from build123d import *

# Parameters (mm, degrees)
SKETCH1_R           = 11
SKETCH1_R_2         = 8
BOSS_EXTRUDE1_DEPTH = 10
SKETCH1_5_R         = 11
BOSS_EXTRUDE3_DEPTH = 5
FILLET2_R           = 1
FILLET3_R           = 1


with BuildPart() as part:
    # Sketch1 → Boss-Extrude1 (new, symmetric)
    with BuildSketch(Plane.XY):
        Circle(SKETCH1_R)
        Circle(SKETCH1_R_2, mode=Mode.SUBTRACT)
    extrude(amount=BOSS_EXTRUDE1_DEPTH, both=True)

    # Sketch1_5 → Boss-Extrude3 (add, symmetric)
    with BuildSketch(Plane.XY):
        with BuildLine():
            ThreePointArc((14.784609691, 12), (13.338075004, 9.857677434), (10.810393031, 10.398817362))
            ThreePointArc((10.810393031, 10.398817362), (10.606601718, 10.606601718), (10.398817362, 10.810393031))
            ThreePointArc((10.398817362, 10.810393031), (9.857677434, 13.338075004), (12, 14.784609691))
            ThreePointArc((12, 14.784609691), (17.795554958, 19.23169542), (15, 25.980762114))
            ThreePointArc((15, 25.980762114), (0, 30), (-15, 25.980762114))
            ThreePointArc((-15, 25.980762114), (-17.795554958, 19.23169542), (-12, 14.784609691))
            ThreePointArc((-12, 14.784609691), (-9.857677434, 13.338075004), (-10.398817362, 10.810393031))
            ThreePointArc((-10.398817362, 10.810393031), (-10.606601718, 10.606601718), (-10.810393031, 10.398817362))
            ThreePointArc((-10.810393031, 10.398817362), (-13.338075004, 9.857677434), (-14.784609691, 12))
            ThreePointArc((-14.784609691, 12), (-19.23169542, 17.795554958), (-25.980762114, 15))
            ThreePointArc((-25.980762114, 15), (-30, 0), (-25.980762114, -15))
            ThreePointArc((-25.980762114, -15), (-19.23169542, -17.795554958), (-14.784609691, -12))
            ThreePointArc((-14.784609691, -12), (-13.338075004, -9.857677434), (-10.810393031, -10.398817362))
            ThreePointArc((-10.810393031, -10.398817362), (-10.606601718, -10.606601718), (-10.398817362, -10.810393031))
            ThreePointArc((-10.398817362, -10.810393031), (-9.857677434, -13.338075004), (-12, -14.784609691))
            ThreePointArc((-12, -14.784609691), (-17.795554958, -19.23169542), (-15, -25.980762114))
            ThreePointArc((-15, -25.980762114), (0, -30), (15, -25.980762114))
            ThreePointArc((15, -25.980762114), (17.795554958, -19.23169542), (12, -14.784609691))
            ThreePointArc((12, -14.784609691), (9.857677434, -13.338075004), (10.398817362, -10.810393031))
            ThreePointArc((10.398817362, -10.810393031), (10.606601718, -10.606601718), (10.810393031, -10.398817362))
            ThreePointArc((10.810393031, -10.398817362), (13.338075004, -9.857677434), (14.784609691, -12))
            ThreePointArc((14.784609691, -12), (19.23169542, -17.795554958), (25.980762114, -15))
            ThreePointArc((25.980762114, -15), (30, 0), (25.980762114, 15))
            ThreePointArc((25.980762114, 15), (19.23169542, 17.795554958), (14.784609691, 12))
        make_face()
        Circle(SKETCH1_5_R, mode=Mode.SUBTRACT)
        with BuildLine():
            ThreePointArc((-13.5, 23.382685902), (-14.598076211, 19.284609691), (-10.5, 18.186533479))
            ThreePointArc((-10.5, 18.186533479), (0, 21), (10.5, 18.186533479))
            ThreePointArc((10.5, 18.186533479), (14.598076211, 19.284609691), (13.5, 23.382685902))
            ThreePointArc((13.5, 23.382685902), (0, 27), (-13.5, 23.382685902))
        make_face(mode=Mode.SUBTRACT)
        with BuildLine():
            ThreePointArc((23.382685902, 13.5), (19.284609691, 14.598076211), (18.186533479, 10.5))
            ThreePointArc((18.186533479, 10.5), (21, 0), (18.186533479, -10.5))
            ThreePointArc((18.186533479, -10.5), (19.284609691, -14.598076211), (23.382685902, -13.5))
            ThreePointArc((23.382685902, -13.5), (27, 0), (23.382685902, 13.5))
        make_face(mode=Mode.SUBTRACT)
        with BuildLine():
            ThreePointArc((13.5, -23.382685902), (14.598076211, -19.284609691), (10.5, -18.186533479))
            ThreePointArc((10.5, -18.186533479), (0, -21), (-10.5, -18.186533479))
            ThreePointArc((-10.5, -18.186533479), (-14.598076211, -19.284609691), (-13.5, -23.382685902))
            ThreePointArc((-13.5, -23.382685902), (0, -27), (13.5, -23.382685902))
        make_face(mode=Mode.SUBTRACT)
        with BuildLine():
            ThreePointArc((-23.382685902, -13.5), (-19.284609691, -14.598076211), (-18.186533479, -10.5))
            ThreePointArc((-18.186533479, -10.5), (-21, 0), (-18.186533479, 10.5))
            ThreePointArc((-18.186533479, 10.5), (-19.284609691, 14.598076211), (-23.382685902, 13.5))
            ThreePointArc((-23.382685902, 13.5), (-27, 0), (-23.382685902, -13.5))
        make_face(mode=Mode.SUBTRACT)
    extrude(amount=BOSS_EXTRUDE3_DEPTH, both=True)

    # Fillet2
    fillet2_edges = [part.edges().sort_by_distance(p)[0] for p in [
        (-11, 0, -10),
        (-8, 0, -10),
    ]]
    fillet(fillet2_edges, radius=FILLET2_R)

    # Fillet3
    fillet3_edges = [part.edges().sort_by_distance(p)[0] for p in [
        (-11, 0, -5),
    ]]
    fillet(fillet3_edges, radius=FILLET3_R)


solid = part.part
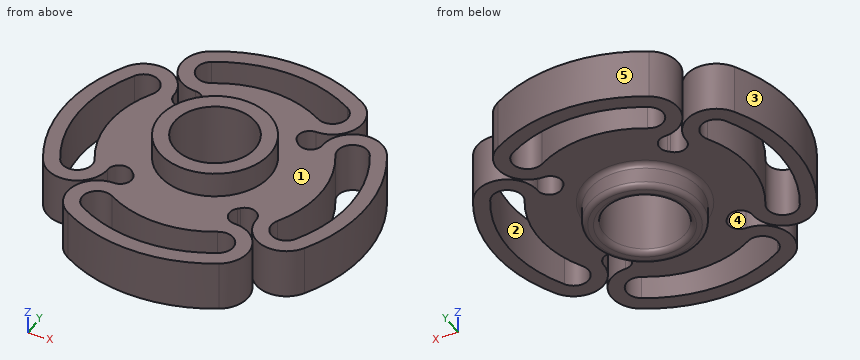
The model under review builds one solid part; all positions refer to its coordinate system, in mm. Face numbers are marked on the shaded views. A direction names the side the tool comes from. Round coordinates to 2 decimals unless told otherwise and drop trailing zeros. Order: outer loops, then holes, each group sorted by start corner. A loop starts at its lowest first (then second) coordinate and runs counter-clockwise, first axis right, second up. Notation, with made-up numbers: (68, 21) - (121, 21) arc R23 cw to (121, 42) - close; hole circle Ø6 at (-35, 36). An arc over 180 degrees is marked (long way). Use one line per item in the form item = value.
Q1. Mouldability with a two-part tool opening along X and no side actions: class the marked faces 3, 4 and 5 as pulls with the +X half, pulls with the -X half, needs draft (parallel to the pull), parting line crosses it, or undercut.
Response values:
face_3 = pulls with the -X half
face_4 = undercut
face_5 = parting line crosses it
Q2. Add section A-A on x = 0. Give the number of separate pieces and of enclosed holes in the cut face, then the cut area to 3 significant figures.
Response values:
separate_pieces = 4
enclosed_holes = 0
area = 380 mm^2
Q3. Clearance check with flat-ended pins moving along their axes: P1, Ø1.5, axis at x = 12, z = 7, coming from the -Y side; P2, Ø8, axis at x = 8.5, z = -6.5, coming from the +Y side; P3, Ø3, axis at x = 6, z = -4, coming from the -Y side; P4, Ø10, axis at y = -14.5, z = 7.5, coming from the +X side. State where each tip first meets the part, or that it passes through.
Response values:
P1 = through
P2 = 29.61
P3 = -29.66
P4 = 28.22
Q4. Add section C-C on x = 16.5. Give the boundary of the cut face in (y, z), then the cut area to 3 significant figures.
Response values:
outline = (-24.75, -5) - (-16.82, -5) - (-16.82, 5) - (-24.75, 5) - close; (-16.2, -5) - (16.2, -5) - (16.2, 5) - (-16.2, 5) - close; (16.82, -5) - (24.75, -5) - (24.75, 5) - (16.82, 5) - close
area = 483 mm^2
Q5. To check wall thickness, follow line 1 (Y direction, x = 0, z = -4); line 2 (Y direction, x = 3, z = 1.75); line 3 (Y direction, x = 9, z = 2.75). State the ranges of each line that lie inside material, in increasing order.
Response values:
line_1 = -30 to -27, -21 to -8, 8 to 21, 27 to 30
line_2 = -29.85 to -26.83, -20.78 to -7.42, 7.42 to 20.78, 26.83 to 29.85
line_3 = -28.62 to -25.46, -18.97 to 18.97, 25.46 to 28.62
Q6. Tool access review of the marked faces 1 and 2: name each direction out of +Z, -Z, +X, -X, +Y, -Y from which nothing blocks a thin tool from reaching the whole face with its end or side.
Response values:
face_1 = +Z
face_2 = +Z, -Z
